```python
from build123d import *

# Parameters (mm, degrees)
SKETCH_1_W          = 100
SKETCH_1_H          = 98.2
EXTRUDE_1_DEPTH     = 5
SKETCH_2_W          = 25
SKETCH_2_H          = 4
EXTRUDE_2_DEPTH     = 23
CHAMFER_1_SIZE      = 5
SKETCH_3_R          = 1.6
CUT_EXTRUDE_1_DEPTH = 100


with BuildPart() as part:
    # 草图1 → 凸台-拉伸1 (new body)
    with BuildSketch(Plane.XY):
        with Locations((-210.886237356, -45)):
            Rectangle(SKETCH_1_W, SKETCH_1_H)
        with BuildLine():
            ThreePointArc((-245.131057565, -22.358440495), (-248.492232664, -20.607289414), (-250.886237356, -23.545446947))
            Line((-250.886237356, -23.545446947), (-250.886237356, -78))
            ThreePointArc((-250.886237356, -78), (-250.0075577, -80.121320344), (-247.886237356, -81))
            Line((-247.886237356, -81), (-224.42573361, -81))
            ThreePointArc((-224.42573361, -81), (-221.919639103, -79.649087724), (-221.670553819, -76.812993548))
            Line((-221.670553819, -76.812993548), (-245.131057565, -22.358440495))
        make_face(mode=Mode.SUBTRACT)
        with BuildLine():
            ThreePointArc((-191.655684006, -33.128922342), (-194.657829236, -31.333405344), (-197.320051564, -33.602618764))
            Line((-197.320051564, -33.602618764), (-208.123721184, -77.279649032))
            ThreePointArc((-208.123721184, -77.279649032), (-207.573803103, -79.849181859), (-205.211489311, -81))
            Line((-205.211489311, -81), (-175.458011282, -81))
            ThreePointArc((-175.458011282, -81), (-172.949810516, -79.645882413), (-172.705875596, -76.805952611))
            Line((-172.705875596, -76.805952611), (-191.655684006, -33.128922342))
        make_face(mode=Mode.SUBTRACT)
        with BuildLine():
            ThreePointArc((-176.638373042, -42.617387799), (-173.276486201, -44.360720795), (-170.886237356, -41.42334041))
            Line((-170.886237356, -41.42334041), (-170.886237356, -12))
            ThreePointArc((-170.886237356, -12), (-171.764917013, -9.878679656), (-173.886237356, -9))
            Line((-173.886237356, -9), (-186.651909841, -9))
            ThreePointArc((-186.651909841, -9), (-189.160110607, -10.354117587), (-189.404045527, -13.194047389))
            Line((-189.404045527, -13.194047389), (-176.638373042, -42.617387799))
        make_face(mode=Mode.SUBTRACT)
        with BuildLine():
            Line((-203.040454286, -12.717792993), (-213.768880163, -56.2546336))
            ThreePointArc((-213.768880163, -56.2546336), (-216.43424337, -58.526613784), (-219.43692336, -56.723847059))
            Line((-219.43692336, -56.723847059), (-238.193779397, -13.187006452))
            ThreePointArc((-238.193779397, -13.187006452), (-237.944694112, -10.350912276), (-235.438599605, -9))
            Line((-235.438599605, -9), (-205.953317692, -9))
            ThreePointArc((-205.953317692, -9), (-203.591816159, -10.149780956), (-203.040454286, -12.717792993))
        make_face(mode=Mode.SUBTRACT)
    extrude(amount=EXTRUDE_1_DEPTH)

    # 草图2 → 凸台-拉伸2 (add)
    with BuildSketch(Plane(origin=(0, 0, 0), x_dir=(-1, 0, 0), z_dir=(0, 0, -1))):
        with Locations((248.386237356, 2.1)):
            Rectangle(SKETCH_2_W, SKETCH_2_H)
        with Locations((248.386237356, -7)):
            Rectangle(SKETCH_2_W, SKETCH_2_H)
        with Locations((173.386237356, -7)):
            Rectangle(SKETCH_2_W, SKETCH_2_H)
        with Locations((173.386237356, 2.1)):
            Rectangle(SKETCH_2_W, SKETCH_2_H)
        with Locations((173.386237356, -92.1)):
            Rectangle(SKETCH_2_W, SKETCH_2_H)
        with Locations((173.386237356, -83)):
            Rectangle(SKETCH_2_W, SKETCH_2_H)
        with Locations((248.386237356, -83)):
            Rectangle(SKETCH_2_W, SKETCH_2_H)
        with Locations((248.386237356, -92.1)):
            Rectangle(SKETCH_2_W, SKETCH_2_H)
    extrude(amount=EXTRUDE_2_DEPTH)

    # 倒角1
    chamfer_1_edges = [part.edges().sort_by_distance(p)[0] for p in [
        (-160.886237356, -7, -23),
        (-160.886237356, 2.1, -23),
        (-160.886237356, -92.1, -23),
        (-160.886237356, -83, -23),
        (-260.886237356, -83, -23),
        (-260.886237356, -92.1, -23),
        (-260.886237356, 2.1, -23),
        (-260.886237356, -7, -23),
    ]]
    chamfer(chamfer_1_edges, length=CHAMFER_1_SIZE)

    # 草图3 → 切除-拉伸1 (cut)
    with BuildSketch(Plane(origin=(0, 4.1, 0), x_dir=(1, 0, 0), z_dir=(0, 1, 0))):
        with Locations(Location((-252.886237356, 18, 0), (0, 0, 270))):
            Circle(SKETCH_3_R)
        with Locations(Location((-240.886237356, 18, 0), (0, 0, 270))):
            Circle(SKETCH_3_R)
        with Locations(Location((-180.886237356, 18, 0), (0, 0, 180))):
            Circle(SKETCH_3_R)
        with Locations(Location((-168.886237356, 18, 0), (0, 0, 180))):
            Circle(SKETCH_3_R)
    extrude(amount=-CUT_EXTRUDE_1_DEPTH, mode=Mode.SUBTRACT)


solid = part.part
```
For this review, take the finished solid that the model builds, in its own axes (mm). A direction names the side the tool comes from. Give positions to 0.01 mm unless a question says otherwise; leave off trailing zeros. Order: outer loops, then holes, each group sorted by start corner. A loop starts at its lowest first (then second) coordinate and runs counter-clockwise, first axis right, second up.
1) Take a section at C-C (y = -60). Give the boundary of the cut face in (x, z), then the cut area to 3 significant figures.
2) For faces 5 (the face through (-235.886, 2, -11)), 6 (the face through (-203.615, -10.12, 2.465)), 7 (the face through (-258.351, -83.028, -20.535)), 8 (the face through (-242.448, -92.072, -18.347)), 9 (the face through (-173, 0.1, -11)), list the 3-axis set-ups (+Z, -Z, +X, -X, +Y, -Y) from which the entire face can be reached by the end or side of a thin tool; tool diameter is ignored.
3) Take a section at A-A (z = -4.5). State how many separate pieces and enclosed holes the cut face has, then the cut area to 3 significant figures.
4) Take a section at B-B (x = -227.5). Give the boundary of the cut face in (y, z).
5) Take a section at D-D (y = -7). Give the boundary of the cut face in (x, z).
6) Insertion check: pin 1 (1.9 mm diameter, centred on x = -240.89, z = -18, fed in from -Y); pin 2 (4 mm diameter, centred on x = -180.89, z = -18, fed in from -Y). Each pin has a flat end and moves straight along its axis. Give the tip position at first contact, or say it passes through.
7) Wall thickness on line 1 (Y direction, x = -167, z = -2.5); line 2 (Y direction, x = -235, z = 2.75); line 3 (Z direction, x = -234, y = -47.5): over which ranges is each line inside the solid? List them lowest first.
8) The part is to be moulded in two halves that separate along X. For faces 1 (the face through (-246, -92, -23)), 2 (the face through (-171.742, -9.902, 2.465)), 3 (the face through (-170.886, -27, 2)), 4 (the face through (-258.421, 2.072, -20.465)), say which applies: released by +X, released by -X, zero draft, split by the parting line, or undercut.
Derived:
1. outline: (-260.89, 0) - (-250.89, 0) - (-250.89, 5) - (-260.89, 5) - close; (-228.91, 0) - (-203.85, 0) - (-203.85, 5) - (-228.91, 5) - close; (-180, 0) - (-160.89, 0) - (-160.89, 5) - (-180, 5) - close
1. area: 271 mm2
2. face 5: -Z, +Y, -Y
2. face 6: +Z, -Z
2. face 7: -Z, -X, +Y, -Y
2. face 8: +Y, -Y
2. face 9: -Z, +X, -X
3. separate pieces: 8
3. enclosed holes: 0
3. area: 800 mm2
4. outline: (-94.1, 0) - (-81, 0) - (-81, 5) - (-94.1, 5) - close; (-63.28, 0) - (-38.01, 0) - (-38.01, 5) - (-63.28, 5) - close; (-9, 0) - (4.1, 0) - (4.1, 5) - (-9, 5) - close
5. outline: (-260.89, -18) - (-255.89, -23) - (-235.89, -23) - (-235.89, 0) - (-185.89, 0) - (-185.89, -23) - (-165.89, -23) - (-160.89, -18) - (-160.89, 5) - (-260.89, 5) - close; hole circle Ø3.2 at (-252.89, -18); hole circle Ø3.2 at (-240.89, -18); hole circle Ø3.2 at (-180.89, -18); hole circle Ø3.2 at (-168.89, -18)
6. pin 1: passes through
6. pin 2: stops at y = -94.1
7. line 1: y = -94.1 to -90.1, -85 to -81, -9 to -5, 0.1 to 4.1
7. line 2: y = -94.1 to -81, -45.87 to -20.6, -9 to 4.1
7. line 3: z = 0 to 5
8. face 1: zero draft
8. face 2: undercut
8. face 3: undercut
8. face 4: released by -X
